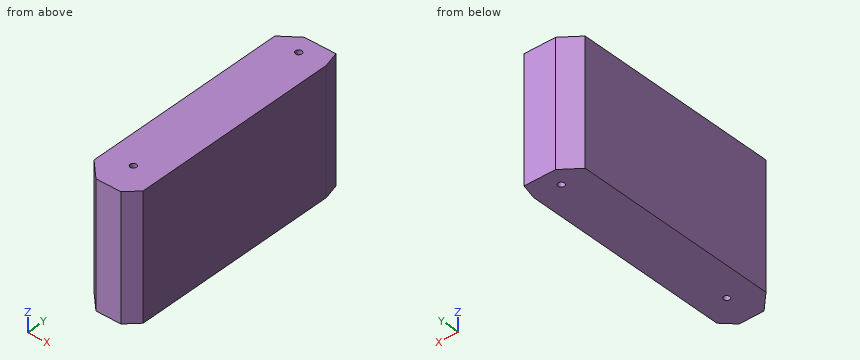
Autodesk Inventor part; units mm, degrees
ref_plane "YZ Plane" through (0, 0, 0) normal (1, 0, 0) x (0, 1, 0)
ref_plane "XZ Plane" through (0, 0, 0) normal (0, 1, 0) x (-1, 0, 0)
ref_plane "XY Plane" through (0, 0, 0) normal (0, 0, 1) x (1, 0, 0)
sketch "Эскиз1" plane through (0, 0, 0) normal (0, 0, 1) x (1, 0, 0)
  line L0 (29.9018, -80.1068) -> (83.774, -134.8208)
  line L1 (83.774, -134.8208) -> (164.0232, -134.8208)
  line L2 (164.0232, -134.8208) -> (202.5632, -96.8737)
  line L3 (202.5632, -96.8737) -> (202.5632, 92.1914)
  line L4 (202.5632, 92.1914) -> (202.5632, 579.95)
  line L5 (202.5632, 579.95) -> (189.081, 631.379)
  line L6 (189.081, 631.379) -> (87.3973, 631.379)
  line L7 (87.3973, 631.379) -> (29.9018, 588.3315)
  line L8 (29.9018, 588.3315) -> (29.9018, -80.1068)
  point P0 (0, 0)
extrude "Выдавливание1" add sketch "Эскиз1" along normal blind 400
sketch "Эскиз2" plane through (0, 0, 0) normal (0, 0, -1) x (-1, 0, 0)
  circle A0 centre (-117.324, -35.3961) radius 10
  circle A1 centre (-117.324, 576.1543) radius 10
  point P0 (0, 0)
  dimension "d2" = 20
  dimension "d3" = 20
extrude "Выдавливание2" cut sketch "Эскиз2" against normal through all
properties part number "Тело"
Verification items for the finished model (mm, model axes). Give positions to 0.01 mm unless a question says otherwise; leave off trailing zeros. Loops run counter-clockwise (first coordinate to the right, second up) from the corner with the lowest first, then second, coordinate; pieces in that order, holes last.
1) Sectioned sample at C-C, the plane x = 44. Enter the section's corners in (y, z).
2) Depth check by flat-ended pin: pin 1 Ø3 at (x, z) = (58, 54) entering from -Y. Enter the tip coordinate at first touch or a pass-through.
3) Thickness scan on line 1 along Y through (x, z) = (126.5, 87); line 2 along Y through (x, z) = (180, 339); line 3 along Y through (x, z) = (76.5, 132). Record the ranges inside material, lowest first.
4) Sectioned sample at A-A, the plane x = 118. Enter the section's corners in (y, z), then the cut area to 3 significant figures.
5) Sectioned sample at B-B, the plane z = 298. Enter the section's corners in (x, y), then the cut area to 3 significant figures.
Answers:
1. outline: (-94.43, 0) - (598.89, 0) - (598.89, 400) - (-94.43, 400) - close
2. pin 1: stops at y = -110.17
3. line 1: y = -134.82 to -39.37, -31.42 to 572.18, 580.13 to 631.38
3. line 2: y = -119.09 to 631.38
3. line 3: y = -127.43 to 623.22
4. outline: (-134.82, 0) - (-45.37, 0) - (-45.37, 400) - (-134.82, 400) - close; (-25.42, 0) - (566.18, 0) - (566.18, 400) - (-25.42, 400) - close; (586.13, 0) - (631.38, 0) - (631.38, 400) - (586.13, 400) - close
4. area: 291,000 mm2
5. outline: (29.9, -80.11) - (83.77, -134.82) - (164.02, -134.82) - (202.56, -96.87) - (202.56, 579.95) - (189.08, 631.38) - (87.4, 631.38) - (29.9, 588.33) - close; hole circle Ø20 at (117.32, -35.4); hole circle Ø20 at (117.32, 576.15)
5. area: 128,000 mm2
